Design review of the part built by this model. Coordinates are the model's own, in mm. Coordinates: 2 decimals unless noted, no trailing zeros. Order: outer loops, then holes, each group sorted by start corner. A loop starts at its lowest first (then second) coordinate and runs counter-clockwise, first axis right, second up. Notation, with made-up numbers: (22.25, 13) -> (49.25, 13) arc R27 cw to (49.25, 40) -> close; hole circle Ø4 at (45.25, 29). An arc over 180 degrees is marked (long way). Use a Markdown table: item, result. Add a question column.
Q1. Add section D-D (x = -37). State the section outline as (y, z) points, then the cut area to 3 significant figures.
Q2. Add section A-A (y = 0). State the section outline as (x, z) points, then the cut area to 3 significant figures.
Q3. The part is to be moulded in two halves that separate along Y. For faces 1 (the face through (-5.185, 0.571, 1.479)), 2 (the face through (-82, 0, 1)), 3 (the face through (-40, 0, 0)), 4 (the face through (-68.57, 0.45, 1.48)), say which applies: pulls with the +Y half, pulls with the -Y half, needs draft (parallel to the pull), parting line crosses it, or undercut.
Q4. Add section B-B (z = 2.35). State the section outline as (x, y) points.
Q5. Wall thickness on probe 1 along Y at (x, z) = (-37, 1.05); probe 2 along Y at (x, z) = (-7, 1.2); probe 3 along X at (y, z) = (3.5, 2.55): over which ranges is each line inside the solid? List them lowest first.
Q6. Insertion check: pin 1 (1.8 mm diameter, centred on x = -70, y = 0, fed in from -Z). The pin has a flat end and moves straight along its axis. Give the tip position at first contact, or say it passes through.
Q7. Add section C-C (x = -7). State the section outline as (y, z) points.
from build123d import *

# Parameters (mm, degrees)
ESQUISSE1_R        = 1.5
ESQUISSE1_R_2      = 1.902389191
BOSS_EXTRU_1_DEPTH = 3


with BuildPart() as part:
    # Esquisse1 → Boss.-Extru.1 (new body)
    with BuildSketch(Plane.XY):
        with BuildLine():
            Line((-70, 12), (0, 12))
            Line((0, 12), (0, -12))
            Line((0, -12), (-70, -12))
            ThreePointArc((-70, -12), (-82, 0), (-70, 12))
        make_face()
        with Locations((-37, 0)):
            Circle(ESQUISSE1_R, mode=Mode.SUBTRACT)
        with Locations((-70, 0)):
            Circle(ESQUISSE1_R, mode=Mode.SUBTRACT)
        with Locations((-7, 0)):
            Circle(ESQUISSE1_R_2, mode=Mode.SUBTRACT)
    extrude(amount=BOSS_EXTRU_1_DEPTH)


solid = part.part
Established:
| question | item | result |
|---|---|---|
| 1 | outline | (-12, 0) -> (-1.5, 0) -> (-1.5, 3) -> (-12, 3) -> close; (1.5, 0) -> (12, 0) -> (12, 3) -> (1.5, 3) -> close |
| 1 | area | 63.0 mm^2 |
| 2 | outline | (-82, 0) -> (-71.5, 0) -> (-71.5, 3) -> (-82, 3) -> close; (-68.5, 0) -> (-38.5, 0) -> (-38.5, 3) -> (-68.5, 3) -> close; (-35.5, 0) -> (-8.9, 0) -> (-8.9, 3) -> (-35.5, 3) -> close; (-5.1, 0) -> (0, 0) -> (0, 3) -> (-5.1, 3) -> close |
| 2 | area | 217 mm^2 |
| 3 | face 1 | undercut |
| 3 | face 2 | parting line crosses it |
| 3 | face 3 | needs draft |
| 3 | face 4 | undercut |
| 4 | outline | (-70, -12) -> (0, -12) -> (0, 12) -> (-70, 12) arc R12 ccw to start; hole circle Ø3 at (-70, 0); hole circle Ø3 at (-37, 0); hole circle Ø3.8 at (-7, 0) |
| 5 | probe 1 | -12 to -1.5, 1.5 to 12 |
| 5 | probe 2 | -12 to -1.9, 1.9 to 12 |
| 5 | probe 3 | -81.48 to 0 |
| 6 | pin 1 | through |
| 7 | outline | (-12, 0) -> (-1.9, 0) -> (-1.9, 3) -> (-12, 3) -> close; (1.9, 0) -> (12, 0) -> (12, 3) -> (1.9, 3) -> close |
